The drawing under review shows one solid part. Ordinate dimensions are in mm from its lowest x, y, z. Give positions to 0.01 mm unless a question says otherwise; leave off trailing zeros. Loops run counter-clockwise (first coordinate to the right, second up) from the corner with the lowest first, then second, coordinate; pieces in that order, holes last. Notation, with made-up numbers: (42, 38.25) - (48, 38.25) arc R29 cw to (48, 65.25) - close; hole circle Ø1 at (-29, -32). An arc over 180 degrees is marked (long way). One line per item, written item: value. Start each with the question number.
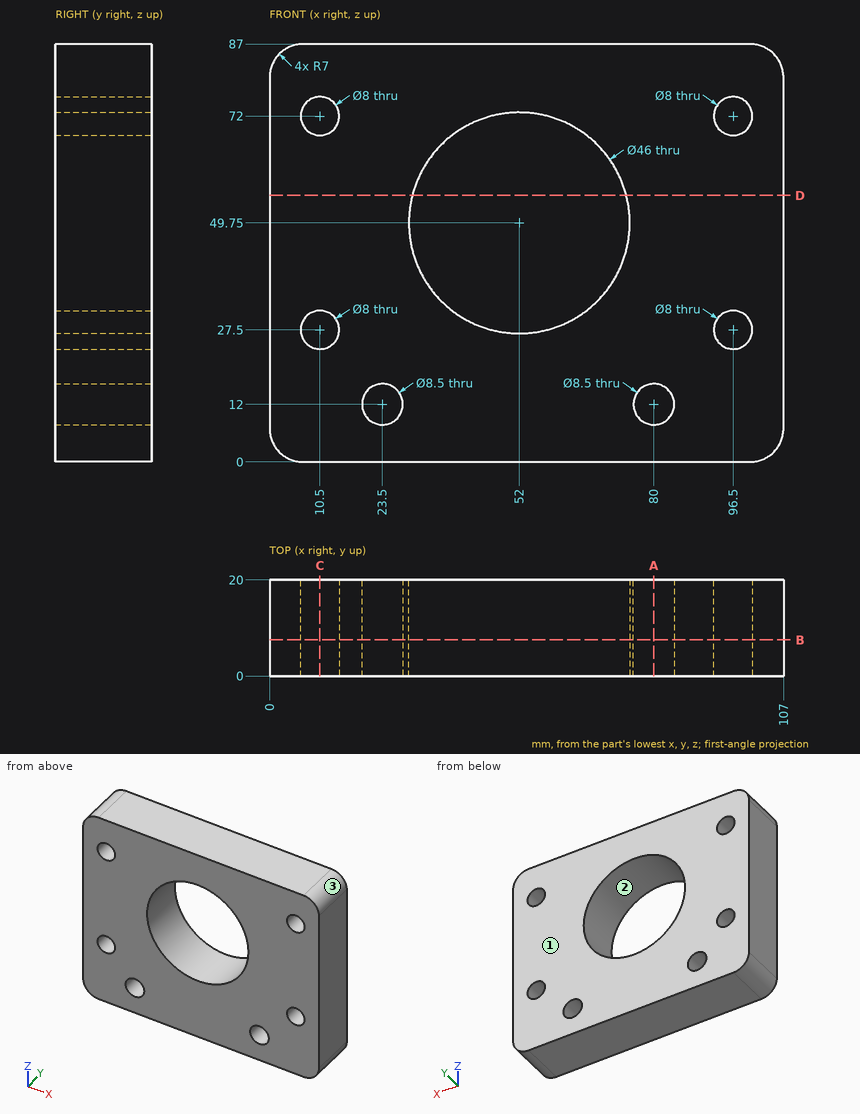
(1) Take a section at D-D on z = 55.5. State the section outline as (x, y) points.
(2) For pin 1 Ø7 at (x, z) = (10.5, 72) entering from -Y, flat-tipped, find the tip position at first contact; note if it passes through.
(3) To check wall thickness, follow L1, parallel to Z at x = 96.5, y = 15; L2, parallel to X at y = 8.75, z = 9; L3, parallel to Z at x = 14, y = 18. State the ranges of each line that lie inside material, in increasing order. Write a range as from..to.
(4) Take a section at C-C on x = 10.5. State the section outline as (y, z) points.
(5) Draft analysis for pull direction Z (two halves, no side actions). For the marked faces 1, 2 and 3, state which applies: pulls with the +Z half, pulls with the -Z half, needs draft (parallel to the pull), parting line crosses it, or undercut.
(6) Take a section at A-A on x = 80. State the section outline as (y, z) points.
(7) Take a section at B-B on y = 7.5. State the section outline as (x, z) points.
Here are the results:
1. outline: (0, 0) - (29.73, 0) - (29.73, 20) - (0, 20) - close; (74.27, 0) - (107, 0) - (107, 20) - (74.27, 20) - close
2. pin 1: through
3. L1: 0..23.5, 31.5..68, 76..87
3. L2: 0..20.49, 26.51..76.99, 83.01..107
3. L3: 0..25.56, 29.44..70.06, 73.94..87
4. outline: (0, 0) - (20, 0) - (20, 23.5) - (0, 23.5) - close; (0, 31.5) - (20, 31.5) - (20, 68) - (0, 68) - close; (0, 76) - (20, 76) - (20, 87) - (0, 87) - close
5. face 1: needs draft
5. face 2: undercut
5. face 3: pulls with the +Z half
6. outline: (0, 0) - (20, 0) - (20, 7.75) - (0, 7.75) - close; (0, 16.25) - (20, 16.25) - (20, 87) - (0, 87) - close
7. outline: (0, 7) arc R7 ccw to (7, 0) - (100, 0) arc R7 ccw to (107, 7) - (107, 80) arc R7 ccw to (100, 87) - (7, 87) arc R7 ccw to (0, 80) - close; hole circle Ø8 at (10.5, 27.5); hole circle Ø8 at (10.5, 72); hole circle Ø8.5 at (23.5, 12); hole circle Ø46 at (52, 49.75); hole circle Ø8.5 at (80, 12); hole circle Ø8 at (96.5, 27.5); hole circle Ø8 at (96.5, 72)
